from build123d import *

# Parameters (mm, degrees)
F0_W     = 13
F0_H     = 13
F1_DEPTH = 95
F3_W     = 13
F3_H     = 2.4
F4_DEPTH = 80
F5_T     = -1.6


with BuildPart() as f1:
    # F0 (on Right) → F1 (new body)
    with BuildSketch(Plane.YZ):
        Rectangle(F0_W, F0_H)
    extrude(amount=F1_DEPTH)

    # F3 (on offset) → F4 (cut)
    with BuildSketch(Plane.YZ.offset(110)):
        Rectangle(F3_W, F3_H)
    extrude(amount=-F4_DEPTH, mode=Mode.SUBTRACT)

    # F5 (hollow: no face is removed)
    offset(amount=F5_T, kind=Kind.INTERSECTION, mode=Mode.SUBTRACT)


solid = f1.part
Can you work these out from the model? Positions are in its coordinate system, mm. A direction names the side the tool comes from. Round coordinates to 2 decimals unless told otherwise and drop trailing zeros. Loops run counter-clockwise (first coordinate to the right, second up) from the corner with the lowest first, then second, coordinate; pieces in that order, holes last. Notation, with made-up numbers: (-13.75, -40) - (14.25, -40) arc R17 cw to (14.25, -19) - close; hole circle Ø3 at (4, -9). An arc over 180 degrees is marked (long way). Use CSV: the item, a comma, the result in double quotes. Start each with the question number.
1) For pin 1 Ø0.7 at (y, z) = (1, -0.5) entering from +X, with a flat end and sliding along its axis, tell me the tip position at first contact or that it passes through.
2) If we section it at B-B on x = 81.5: Write out the boundary of the cut face in (y, z).
3) If we section it at C-C on y = -2.5: Write out the boundary of the cut face in (x, z).
4) Please list where these lines run through material, in increasing order: probe 1 along Z at (x, y) = (66.5, 3.25); probe 2 along Z at (x, y) = (26, -4.5). Write a range as [from, to].
5) For faces 1 (the flat face through (47, 0, 4.9)), 2 (the flat face through (30, 0, 0)), 3 (the flat face through (47, 0, 6.5)), which set-ups out of +Z, -Z, +X, -X, +Y, -Y let a thin tool reach every point of the face, with its end or its side?
6) We'd pull the mould along Y, two halves only. Please class faces 4 (the flat face through (61, 0, -2.8)), 5 (the flat face through (63, 0, -1.2)), 6 (the flat face through (47, -6.5, -2)): released by +Y, released by -Y, zero draft, split by the parting line, or undercut.
7) If we section it at A-A on z = -2: Write out the boundary of the cut face in (x, y).
Geometry results:
1,pin 1,"stops at x = 30"
2,outline,"(-6.5, -6.5) - (6.5, -6.5) - (6.5, -1.2) - (-6.5, -1.2) - close; (-6.5, 1.2) - (6.5, 1.2) - (6.5, 6.5) - (-6.5, 6.5) - close; hole (-4.9, -4.9) - (4.9, -4.9) - (4.9, -2.8) - (-4.9, -2.8) - close; hole (-4.9, 2.8) - (4.9, 2.8) - (4.9, 4.9) - (-4.9, 4.9) - close"
3,outline,"(0, -6.5) - (95, -6.5) - (95, -1.2) - (30, -1.2) - (30, 1.2) - (95, 1.2) - (95, 6.5) - (0, 6.5) - close; hole (1.6, -4.9) - (93.4, -4.9) - (93.4, -2.8) - (28.4, -2.8) - (28.4, 2.8) - (93.4, 2.8) - (93.4, 4.9) - (1.6, 4.9) - close"
4,probe 1,"z = [-6.5, -4.9], [-2.8, -1.2], [1.2, 2.8], [4.9, 6.5]"
4,probe 2,"z = [-6.5, -4.9], [4.9, 6.5]"
5,face 1,"none"
5,face 2,"+X, +Y, -Y"
5,face 3,"+Z, +X, -X, +Y, -Y"
6,face 4,"undercut"
6,face 5,"zero draft"
6,face 6,"released by -Y"
7,outline,"(0, -6.5) - (95, -6.5) - (95, 6.5) - (0, 6.5) - close; hole (1.6, -4.9) - (28.4, -4.9) - (28.4, 4.9) - (1.6, 4.9) - close"
